```python
from build123d import *

# Parameters (mm, degrees)
ESQUISSE1_W             = 140
ESQUISSE1_H             = 15
BOSS_EXTRU_1_DEPTH      = 4
ENL_V_MAT_EXTRU_1_DEPTH = 10
ESQUISSE3_W             = 60
ESQUISSE3_H             = 8.5
ENL_V_MAT_EXTRU_2_DEPTH = 10
CONG_1_R                = 1.5


with BuildPart() as part:
    # Esquisse1 → Boss.-Extru.1 (new body)
    with BuildSketch(Plane.XY):
        with Locations((0, 7.5)):
            Rectangle(ESQUISSE1_W, ESQUISSE1_H)
    extrude(amount=BOSS_EXTRU_1_DEPTH)

    # Esquisse2 → Enlèv. mat.-Extru.1 (cut)
    with BuildSketch(Plane.XY.offset(4)):
        Polygon((-64, 15), (-64, 12), (-67, 12), (-67, 6.5), (-35, 6.5), (-35, 12), (-38, 12), (-38, 15), align=None)
        Polygon((38, 12), (38, 15), (64, 15), (64, 12), (67, 12), (67, 6.5), (35, 6.5), (35, 12), align=None)
    extrude(amount=-ENL_V_MAT_EXTRU_1_DEPTH, mode=Mode.SUBTRACT)

    # Esquisse3 → Enlèv. mat.-Extru.2 (cut)
    with BuildSketch(Plane.XY.offset(4)):
        with Locations((0, 10.75)):
            Rectangle(ESQUISSE3_W, ESQUISSE3_H)
    extrude(amount=-ENL_V_MAT_EXTRU_2_DEPTH, mode=Mode.SUBTRACT)

    # Congé1
    cong_1_edges = [part.edges().sort_by_distance(p)[0] for p in [
        (30, 15, 2),
        (38, 15, 2),
        (64, 15, 2),
        (70, 15, 2),
        (-70, 0, 2),
        (-70, 15, 2),
        (-64, 15, 2),
        (-64, 12, 2),
        (-67, 12, 2),
        (-67, 6.5, 2),
        (-35, 6.5, 2),
        (-35, 12, 2),
        (-38, 12, 2),
        (-38, 15, 2),
        (-30, 15, 2),
        (-30, 6.5, 2),
        (30, 6.5, 2),
        (35, 6.5, 2),
        (67, 6.5, 2),
        (70, 0, 2),
        (64, 12, 2),
        (67, 12, 2),
        (35, 12, 2),
        (38, 12, 2),
    ]]
    fillet(cong_1_edges, radius=CONG_1_R - 0.0001)  # a hair under: the kernel refuses the full size


solid = part.part
```
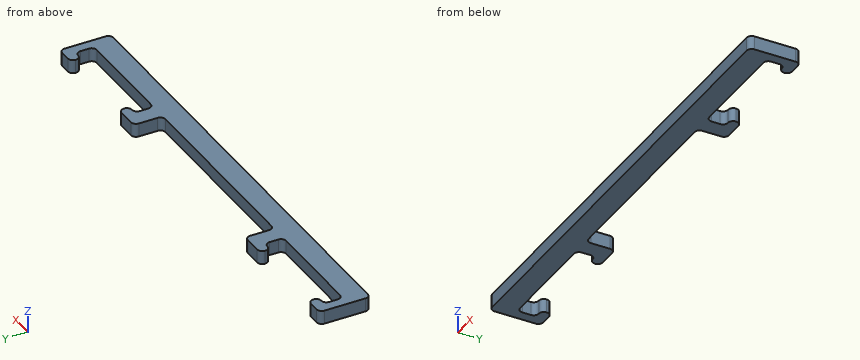
Geometry check sheet. Reference: the model listing, model coordinates, mm. Coordinates: 2 decimals unless noted, no trailing zeros. Loops run counter-clockwise (first coordinate to the right, second up) from the corner with the lowest first, then second, coordinate; pieces in that order, holes last.
Item 1: Sectioned sample at A-A, the plane x = 42. Record the boundary of the cut face in (y, z).
Item 2: Go/stop test with a flat-tipped pin: pin 1 Ø1.2 at (x, z) = (-51.5, 2) entering from +Y. Record where the tip stops, or that it passes through.
Item 3: Thickness scan on line 1 (X direction, y = 9, z = 3.85); line 2 (X direction, y = 13.25, z = 0.95); line 3 (Y direction, x = 11, z = 3.65). Record the ranges inside material, lowest first.
Check result:
1. outline: (0, 0) - (6.5, 0) - (6.5, 4) - (0, 4) - close
2. pin 1: stops at y = 6.5
3. line 1: x = -70 to -67, -35 to -30, 30 to 35, 67 to 70
3. line 2: x = -70 to -64.02, -37.98 to -30, 30 to 37.98, 64.02 to 70
3. line 3: y = 0 to 6.5
